from build123d import *

# Parameters (mm, degrees)
BOSS_EXTRUDE1_DEPTH = 5
BOSS_EXTRUDE2_DEPTH = 3
SKETCH3_W           = 2.803061543
SKETCH3_H           = 5
BOSS_EXTRUDE3_DEPTH = 1
BOSS_EXTRUDE4_DEPTH = 0.5
SKETCH5_W           = 7.386047788
SKETCH5_H           = 39
CHAMFER2_SIZE       = 0.25


with BuildPart() as part:
    # Sketch1 → Boss-Extrude1 (new body, symmetric)
    with BuildSketch(Plane.XY):
        with BuildLine():
            Line((-14.696938457, 34.5), (-14.696938457, 9.5))
            ThreePointArc((-14.696938457, 9.5), (-16.784612343, 4.952452777), (-17.5, 0))
            Line((-17.5, 0), (-42.802853896, 0))
            ThreePointArc((-42.802853896, 0), (-38.211284713, 19.612097715), (-24.644146108, 34.5))
            Line((-24.644146108, 34.5), (-24.644146108, 28.265103266))
            ThreePointArc((-24.644146108, 28.265103266), (-19.916041725, 31.774223547), (-14.696938457, 34.5))
        make_face()
    boss_extrude1 = extrude(amount=BOSS_EXTRUDE1_DEPTH, both=True)

    # Sketch2 → Boss-Extrude2 (add)
    with BuildSketch(Plane.XY.offset(5)):
        Polygon((-26, 0), (-17.5, 0), (-17.5, 2), (-20, 2.577874668), (-20, 5.577874668), (-17.5, 6.155749336), (-17.5, 9.524542718), (-20, 10.102417386), (-20, 13.102417386), (-17.5, 13.680292054), (-17.5, 15), (-17.5, 22), (-26, 22), (-26, 15.5), (-30.001513248, 12.421912886), (-30.001513248, 8.421912886), (-32.5, 6.5), (-32.5, 0), align=None)
    boss_extrude2 = extrude(amount=BOSS_EXTRUDE2_DEPTH)

    # Sketch3 → Boss-Extrude3 (add)
    with BuildSketch(Plane.XY.offset(5)):
        with Locations((-16.098469229, 17.5)):
            Rectangle(SKETCH3_W, SKETCH3_H)
    boss_extrude3 = extrude(amount=BOSS_EXTRUDE3_DEPTH)

    # Sketch4 → Boss-Extrude4 (add)
    with BuildSketch(Plane.XY.offset(5)):
        Polygon((-26, 22), (-18.495062021, 26.599255094), (-17.5, 26.5), (-17.5, 22), align=None)
    boss_extrude4 = extrude(amount=BOSS_EXTRUDE4_DEPTH)

    # Sketch5 → Cut-Revolve1 (revolve, cut)
    with BuildSketch(Plane(origin=(0, 0, 0), x_dir=(0, 0, -1), z_dir=(1, 0, 0))):
        with Locations((-0.102834864, 19.5)):
            Rectangle(SKETCH5_W, SKETCH5_H)
    cut_revolve1 = revolve(axis=Axis((0, 0, 3.795858758), (0, 0, -1)), mode=Mode.SUBTRACT)

    # Mirror1: Boss-Extrude1, Boss-Extrude2, Boss-Extrude3, Boss-Extrude4, Cut-Revolve1 across plane
    add(boss_extrude1.mirror(Plane.ZX))
    add(boss_extrude2.mirror(Plane.ZX))
    add(boss_extrude3.mirror(Plane.ZX))
    add(boss_extrude4.mirror(Plane.ZX))
    add(cut_revolve1.mirror(Plane.ZX), mode=Mode.SUBTRACT)

    # Chamfer2
    chamfer2_edges = [part.edges().sort_by_distance(p)[0] for p in [
        (-20, -11.602417386, 8),
        (-18.75, -9.813480052, 8),
        (-17.5, -7.840146027, 8),
        (-18.75, -5.866812002, 8),
        (-31.250756624, -7.460956443, 8),
        (-30.001513248, -10.421912886, 8),
        (-28.000756624, -13.960956443, 8),
        (-21.75, -22, 8),
        (-18.75, -13.39135472, 8),
        (-20, -4.077874668, 8),
        (-18.75, -2.288937334, 8),
        (-26, -18.75, 8),
        (-17.5, -17.840146027, 8),
        (-17.5, 17.840146027, 8),
        (-26, 18.75, 8),
        (-18.75, 2.288937334, 8),
        (-20, 4.077874668, 8),
        (-20, 11.602417386, 8),
        (-18.75, 13.39135472, 8),
        (-21.75, 22, 8),
        (-28.000756624, 13.960956443, 8),
        (-30.001513248, 10.421912886, 8),
        (-31.250756624, 7.460956443, 8),
        (-32.5, 0, 8),
        (-17.5, 0, 8),
        (-18.75, 5.866812002, 8),
        (-17.5, 7.840146027, 8),
        (-18.75, 9.813480052, 8),
    ]]
    chamfer(chamfer2_edges, length=CHAMFER2_SIZE)


solid = part.part
CAD build for the part. Positions are in the model's coordinates, mm. A direction names the side the tool comes from. Round coordinates to 2 decimals unless told otherwise and drop trailing zeros. Write each loop counter-clockwise with the first axis right and the second up, starting at its lowest first coordinate (ties: lowest second). Pieces come first, ordered by that corner, then holes. Notation, with made-up numbers: M 23.5,-18 L 57.5,-18 A12 ccw 57.5,-10 Z; hole C 66,13.25 d11. An arc over 180 degrees is marked long. Put each result on its own line as item: value. Start each with the question number.
1) Pull direction Y, two halves, no side cores. Call faces 1 (the flat face through (-27.973, -13.983, 6.356)), 2 (the flat face through (-20, 4, 6)), 3 (the flat face through (-18.732, 2.285, 6.356)), 4 (the flat face through (-30.002, 10, 6)): pulls with the +Y half, pulls with the -Y half, needs draft (parallel to the pull), parting line crosses it, or undercut.
2) 3-axis set-ups, long thin cutter, end or side, ignore diameter. For faces 5 (the flat face through (-32.5, 0, 6)), 6 (the flat face through (-18.7, 9.8, 6.4)), 7 (the flat face through (-22.3, -24.267, 5.246)), 8 (the flat face through (-24, 0, 3.796)): which of +Z, -Z, +X, -X, +Y, -Y reach the whole face in a straight line?
3) Saw through at D-D, the plane z = -1.5. Write the cut outline in (x, y), and give its area (3 significant figures).
4) Saw through at C-C, the plane x = -23.5. Write the cut outline in (y, z), and give its area (3 significant figures).
5) Saw through at B-B, the plane y = 18.5. Write the cut outline in (x, z), and give its area (3 significant figures).
6) Pin check, flat tips, straight feed: pin 1 Ø4 at (x, z) = (-32.5, 3) entering from -Y; pin 2 Ø6 at (x, y) = (-16, 8) entering from +Z; pin 3 Ø1.4 at (y, z) = (1, 6.5) entering from -X; pin 4 Ø1.4 at (y, z) = (-19, 6) entering from -X. Stop position of each tip, or through.
7) Drill centre lines: probe 1 along Z at (x, y) = (-21.75, -28.5); probe 2 along Z at (x, y) = (-29.5, -28.5); probe 3 along Y at (x, z) = (-35, 1.25). Where is each one in solid material? Low to high. Write a range as [from, to].
8) Saw through at A-A, the plane x = -27. Write the cut outline in (y, z), and give its area (3 significant figures).
Resolved:
1. face 1: pulls with the -Y half
1. face 2: undercut
1. face 3: undercut
1. face 4: needs draft
2. face 5: +Z, -X, +Y, -Y
2. face 6: +Z, +X
2. face 7: +Z, -X, -Y
2. face 8: +X
3. outline: M -42.8,0 A40 ccw -24.64,-34.5 L -24.64,-30.23 A39 cw -24.64,30.23 L -24.64,34.5 A40 ccw Z
3. area: 290 mm²
4. outline: M -29.22,-5 L 29.22,-5 L 29.22,-3.59 L -29.22,-3.59 Z; M -29.22,3.8 L 29.22,3.8 L 29.22,5 L 23.53,5 L 23.53,5.5 L 22,5.5 L 22,7.75 L 21.75,8 L -21.75,8 L -22,7.75 L -22,5.5 L -23.53,5.5 L -23.53,5 L -29.22,5 Z
4. area: 286 mm²
5. outline: M -38.77,-5 L -14.7,-5 L -14.7,-3.59 L -34.33,-3.59 L -34.33,3.8 L -14.7,3.8 L -14.7,6 L -17.5,6 L -17.5,7.75 L -17.75,8 L -25.75,8 L -26,7.75 L -26,5 L -38.77,5 Z
5. area: 124 mm²
6. pin 1: y = -29.85
6. pin 2: z = 8
6. pin 3: x = -32.5
6. pin 4: x = -26
7. probe 1: [-5, -3.59], [3.8, 5]
7. probe 2: [-5, 5]
7. probe 3: [-24.73, -17.2], [17.2, 24.73]
8. outline: M -32.84,-5 L 32.84,-5 L 32.84,5 L 14.73,5 L 14.73,7.75 L 14.42,8 L -14.42,8 L -14.73,7.75 L -14.73,5 L -32.84,5 Z; hole M -28.14,-3.59 L 28.14,-3.59 L 28.14,3.8 L -28.14,3.8 Z
8. area: 329 mm²
